Could you check a few things on this model? Use its own coordinates, in mm. A direction names the side the tool comes from. Round coordinates to 2 decimals unless told otherwise and drop trailing zeros. Order: outer loops, then holes, each group sorted by start corner. A loop starts at its lowest first (then second) coordinate and runs counter-clockwise, first axis right, second up. Notation, with made-up numbers: (-7.75, -24.75) -> (1.25, -24.75) arc R7 cw to (1.25, -16.75) -> close; hole circle Ø5 at (20.5, -33). An arc over 180 degrees is marked (long way). Put each result on its own line as item: value. Start each with the question number.
from build123d import *

# Parameters (mm, degrees)
SKETCH_R      = 27.5
SKETCH_R_2    = 22.5
SKETCH_R_3    = 1
PAD_DEPTH     = 10
SKETCH001_R   = 22.5
SKETCH001_R_2 = 14
PAD001_DEPTH  = 4
SKETCH004_R   = 14
SKETCH004_R_2 = 13.5
PAD004_DEPTH  = 16


with BuildPart() as part:
    # Sketch → Pad (new body)
    with BuildSketch(Plane.XY):
        Circle(SKETCH_R)
        Circle(SKETCH_R_2, mode=Mode.SUBTRACT)
        with Locations((0, 25)):
            Circle(SKETCH_R_3, mode=Mode.SUBTRACT)
        with Locations((-21.650635, -12.5)):
            Circle(SKETCH_R_3, mode=Mode.SUBTRACT)
        with Locations((21.650635, -12.5)):
            Circle(SKETCH_R_3, mode=Mode.SUBTRACT)
    extrude(amount=PAD_DEPTH)

    # Sketch001 → Pad001 (join)
    with BuildSketch(Plane.XY):
        Circle(SKETCH001_R)
        Circle(SKETCH001_R_2, mode=Mode.SUBTRACT)
    extrude(amount=PAD001_DEPTH)

    # Sketch004 → Pad004 (join)
    with BuildSketch(Plane.XY):
        Circle(SKETCH004_R)
        Circle(SKETCH004_R_2, mode=Mode.SUBTRACT)
    extrude(amount=PAD004_DEPTH)


solid = part.part
1. I need wall thicknesses on L1, parallel to Y at x = 0, z = 8.75; L2, parallel to Y at x = 0, z = 12.25; L3, parallel to Y at x = -9, z = 9.5. Which ranges of each line are inside material? Lowest first, please.
2. If we section it at D-D, the plane x = -7: Please give me the cut outline in (y, z).
3. If we section it at C-C, the plane y = -1: Please give me the cut outline in (x, z).
4. For pin 1 Ø5 at (x, z) = (6, 4) entering from -Y; pin 2 Ø8 at (x, z) = (-10.5, 10.5) entering from +Y; pin 3 Ø1.5 at (x, z) = (0.5, 6) entering from -Y, each with a flat end and sliding along its axis, tell me the tip position at first contact or that it passes through.
5. If we section it at B-B, the plane z = 3.25: Please give me the cut outline in (x, y), then the cut area to 3 significant figures.
6. Which directions (+Z, -Z, +X, -X, +Y, -Y) give clear straight access to the entire face, cutting with the end or side of a thin tool? Please do faces 1 (the face through (-22.65, -12.46, 4.93)), 2 (the face through (-10.32, -9.69, 4)).
7. Thinking about a two-plate mould opening in X: for faces 3 (the face through (-10.3, -20.2, 10)), 4 (the face through (12.932, -5.362, 9.916)), 5 (the face through (-5.961, -26.846, 4.93)), which applies, +X half, -X half, draft (parallel to the pull), parting line (faces both ways), or undercut?
8. If we section it at A-A, the plane x = 0: Please give me the cut outline in (y, z).
Results below:
1. L1: -27.5 to -22.5, -14 to -13.5, 13.5 to 14, 22.5 to 24, 26 to 27.5
1. L2: -14 to -13.5, 13.5 to 14
1. L3: -25.99 to -20.62, -10.72 to -10.06, 10.06 to 10.72, 20.62 to 25.99
2. outline: (-26.59, 0) -> (-11.54, 0) -> (-11.54, 16) -> (-12.12, 16) -> (-12.12, 4) -> (-21.38, 4) -> (-21.38, 10) -> (-26.59, 10) -> close; (11.54, 0) -> (26.59, 0) -> (26.59, 10) -> (21.38, 10) -> (21.38, 4) -> (12.12, 4) -> (12.12, 16) -> (11.54, 16) -> close
3. outline: (-27.48, 0) -> (-13.46, 0) -> (-13.46, 16) -> (-13.96, 16) -> (-13.96, 4) -> (-22.48, 4) -> (-22.48, 10) -> (-27.48, 10) -> close; (13.46, 0) -> (27.48, 0) -> (27.48, 10) -> (22.48, 10) -> (22.48, 4) -> (13.96, 4) -> (13.96, 16) -> (13.46, 16) -> close
4. pin 1: y = -27.28
4. pin 2: y = 26.71
4. pin 3: y = -27.5
5. outline: circle Ø55 at (0, 0); hole circle Ø2 at (-21.65, -12.5); hole circle Ø27 at (0, 0); hole circle Ø2 at (0, 25); hole circle Ø2 at (21.65, -12.5)
5. area: 1,790 mm2
6. face 1: +Z, -Z
6. face 2: +Z
7. face 3: draft
7. face 4: undercut
7. face 5: parting line
8. outline: (-27.5, 0) -> (-13.5, 0) -> (-13.5, 16) -> (-14, 16) -> (-14, 4) -> (-22.5, 4) -> (-22.5, 10) -> (-27.5, 10) -> close; (13.5, 0) -> (24, 0) -> (24, 10) -> (22.5, 10) -> (22.5, 4) -> (14, 4) -> (14, 16) -> (13.5, 16) -> close; (26, 0) -> (27.5, 0) -> (27.5, 10) -> (26, 10) -> close
